Could you check a few things on this model? Use its own coordinates, in mm. A direction names the side the tool comes from. Coordinates: 2 decimals unless noted, no trailing zeros. Order: outer loops, then holes, each group sorted by start corner. A loop starts at its lowest first (then second) coordinate and runs counter-clockwise, first axis right, second up. Notation, with made-up numbers: (53, 22.5) -> (76, 22.5) arc R29 cw to (76, 57.5) -> close; hole circle Ø2 at (87.5, 36). An arc over 180 degrees is marked (long way). Return JSON: item names as keys, results as strings. Group by question number.
from build123d import *

# Parameters (mm, degrees)
F0_W    = 6
F0_H    = 22.5
F2_SIZE = 1.5
F3_R    = 1.49999


# Not quite as in the source:
# - a fillet or chamfer is up to 0.001 mm smaller than in the source, because OpenCascade refuses the exact size


with BuildPart() as f1:
    # F0 (on Front) → F1 (revolve)
    with BuildSketch(Plane.XZ):
        with Locations((3, 11.25)):
            Rectangle(F0_W, F0_H)
        Polygon((6, 0), (0, 0), (0, -3.75), (7.5, -3.75), (7.5, 0), align=None)
    revolve(axis=Axis((0, 0, 8.5798527999), (0, 0, -1)))

    # F2
    f2_edges = [f1.edges().sort_by_distance(p)[0] for p in [
        (-6, 0, 22.5),
    ]]
    chamfer(f2_edges, length=F2_SIZE)

    # F3 (radius 1.5 in the source; OpenCascade refuses exactly that, so slightly less here)
    f3_edges = [f1.edges().sort_by_distance(p)[0] for p in [
        (-6, 0, 0),
    ]]
    fillet(f3_edges, radius=F3_R)


solid = f1.part
Q1. I want a section at C-C on z = -1.5. Please give me the cut outline in (x, y).
Q2. I need wall thicknesses on line 1 along Z through (x, y) = (4.25, 3.5); line 2 along X through (y, z) = (5.5, 7.75); line 3 along Z through (x, y) = (0.25, -5.75). Which ranges of each line are inside material? Lowest first, please. Write a range as from..to.
Q3. I'm going to push flat-ended pins straight in: pin 1 Ø5 at (x, z) = (2.5, 14.5) entering from +Y; pin 2 Ø5 at (x, z) = (-5, 14.5) entering from -Y; pin 3 Ø3 at (x, y) = (-6, -1.5) entering from +Z. Where does each tip first touch, or does it pass through?
Q4. On a 3-axis mill with a long thin cutter (end or side, diameter ignored), from which of +Z, -Z, +X, -X, +Y, -Y can I reach the whole of each face in a straight line? I mean faces 1 (the cylindrical face through (-7.493, -0.33, -1.849)), 2 (the cylindrical face through (-6, 0, 11)). Say none if no direction works.
Q5. I want a section at D-D on z = 15.5. Please give me the cut outline in (x, y).
Response values:
{
 "1": {"outline": "circle Ø15 at (0, 0)"},
 "2": {"line 1": "z = -3.75..21.49", "line 2": "x = -2.4..2.4", "line 3": "z = -3.75..21.24"},
 "3": {"pin 1": "stops at y = 6", "pin 2": "stops at y = -5.45", "pin 3": "stops at z = 22.32"},
 "4": {"face 1": "+Z, -Z", "face 2": "+Z"},
 "5": {"outline": "circle Ø12 at (0, 0)"}
}
